The listing builds one solid part. Answer for the finished solid, in the listing's coordinates (mm). Face numbers are marked on the shaded views. A direction names the side the tool comes from. Round coordinates to 2 decimals unless told otherwise and drop trailing zeros. Write each loop counter-clockwise with the first axis right and the second up, starting at its lowest first coordinate (ties: lowest second). Pieces come first, ordered by that corner, then holes. Notation, with made-up numbers: (49.5, 31) - (105.5, 31) arc R21 cw to (105.5, 62) - close; hole circle Ø1 at (-26.5, -3). An arc over 180 degrees is marked (long way). Return JSON: item names as keys, results as strings. Group by question number.
(1) Determine the mould class of the marked faces 1, 2, 3 and 4 for opening direction Y: +Y half, -Y half, draft (parallel to the pull), parting line (faces both ways), or undercut.
(2) Section A-A, the plane x = 27.5 is taken. Write down the section's boundary in (y, z).
(3) Section D-D, the plane z = 12.5 is taken. Write down the section's boundary in (x, y), then the cut area to 3 significant figures.
(4) Find the intervals of material crossed by line 1 along Y through (x, z) = (2.35, 19.8); line 2 along Y through (x, z) = (13.7, 71.9); line 3 along X through (y, z) = (17.5, 18), in increasing order. Write a range as [from, to].
(5) Section B-B, the plane z = 56.4 is taken. Write down the section's boundary in (x, y).
(6) Section C-C, the plane x = 18 is taken. Write down the section's boundary in (y, z), then the cut area to 3 significant figures.
(7) Each of these flat-tipped pins is pushed along its axis until it touches: pin 1 (2.5 mm diameter, centred on y = 11.5, z = 71.9, fed in from -X); pin 2 (5.5 mm diameter, centred on y = 11.5, z = 71.9, fed in from -X); pin 3 (1.8 mm diameter, centred on y = 10, z = 71, fed in from +X). Where does it stop, or does it pass through?
(8) Which of the six approach directions +Z, -Z, +X, -X, +Y, -Y give full straight-line access (tool end or side, diameter ignored) to the marked faces 5, 6 and 7?
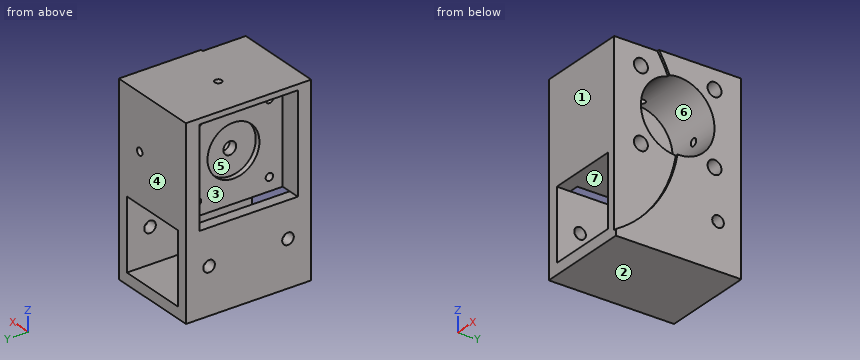
Autodesk Inventor part; units mm, degrees
ref_plane "YZ Plane" through (0, 0, 0) normal (1, 0, 0) x (0, 1, 0)
ref_plane "XZ Plane" through (0, 0, 0) normal (0, 1, 0) x (-1, 0, 0)
ref_plane "XY Plane" through (0, 0, 0) normal (0, 0, 1) x (1, 0, 0)
sketch "Sketch1" plane through (0, 0, 0) normal (0, 0, 1) x (1, 0, 0)
  line L0 (0, 0) -> (40, 0)
  line L1 (40, 0) -> (40, 54)
  line L2 (40, 54) -> (0, 54)
  line L3 (0, 54) -> (0, 0)
  dimension "d0" = 40
  dimension "d1" = 54
extrude "Extrusion1" add sketch "Sketch1" along normal blind 80
sketch "Sketch3" plane through (0, 0, 0) normal (0, -1, 0) x (1, 0, 0)
  line L0 (4.8, 4.8) -> (35.2, 4.8)
  line L1 (35.2, 4.8) -> (35.2, 35.2)
  line L2 (35.2, 35.2) -> (4.8, 35.2)
  line L3 (4.8, 35.2) -> (4.8, 4.8)
  line L4 (0, 0) -> (40, 0)
  line L5 (0, 0) -> (0, 80)
  dimension "d7" = 30.4
  dimension "d8" = 30.4
  dimension "d9" = 4.8
  dimension "d10" = 4.8
extrude "Extrusion2" cut sketch "Sketch3" against normal blind 80
sketch "Sketch4" plane through (0, 0, 0) normal (-1, 0, 0) x (0, 0, 1)
  line L0 (35.2, 0) -> (35.2, 54)
  line L1 (35.2, 5.8) -> (77.6, 5.8)
  line L2 (77.6, 5.8) -> (77.6, 48.2)
  line L3 (77.6, 48.2) -> (35.2, 48.2)
  line L4 (35.2, 48.2) -> (35.2, 5.8)
  line L5 (0, 0) -> (80, 0)
  point P0 (35.2, 48.2)
  dimension "d13" = 42.4
  dimension "d14" = 42.4
  dimension "d15" = 5.8
extrude "Extrusion3" cut sketch "Sketch4" against normal blind 9
sketch "Sketch5" plane through (9, 0, 0) normal (-1, 0, 0) x (0, 0, 1)
  circle A0 centre (71.9, 42.5) radius 1.6
  circle A1 centre (71.9, 11.5) radius 1.6
  circle A2 centre (40.9, 42.5) radius 1.6
  circle A3 centre (40.9, 11.5) radius 1.6
  circle A4 centre (56.4, 27) radius 2.75
  line L0 (71.9, 42.5) -> (71.9, 11.5)
  line L1 (71.9, 11.5) -> (40.9, 11.5)
  line L2 (40.9, 11.5) -> (40.9, 42.5)
  line L3 (40.9, 42.5) -> (71.9, 42.5)
  line L4 (77.6, 48.2) -> (77.6, 5.8)
  line L5 (35.2, 48.2) -> (77.6, 48.2)
  point P0 (0, 0)
  dimension "d18" = 3.2
  dimension "d19" = 31
  dimension "d20" = 31
  dimension "d21" = 5.7
  dimension "d22" = 5.7
  dimension "d23" = 15.5
  dimension "d24" = 15.5
  dimension "d25" = 5.5
extrude "Extrusion4" cut sketch "Sketch5" against normal blind 40 contours A0 L0 L3 | L3 L0 A0 | L3 L2 A2 | A2 L2 L3 | L0 L1 A1 | A1 L1 L0 | L2 L1 A3 | A3 L1 L2 | A4
sketch "Sketch7" plane through (40, 0, 0) normal (1, 0, 0) x (0, 0, -1)
  circle A0 centre (-56.4, 27) radius 15.5
  circle A1 centre (-56.4, 27) radius 2.75
  circle A2 centre (-71.9, 11.5) radius 1.6
  circle A3 centre (-71.9, 11.5) radius 3
  circle A4 centre (-40.9, 11.5) radius 1.6
  circle A5 centre (-40.9, 11.5) radius 3
  circle A6 centre (-40.9, 42.5) radius 1.6
  circle A7 centre (-40.9, 42.5) radius 3
  circle A8 centre (-71.9, 42.5) radius 1.6
  circle A9 centre (-71.9, 42.5) radius 3
  point P0 (0, 0)
  point P1 (-72.8896, 14.2541)
  point P2 (-68.9459, 10.3104)
  point P3 (-43.4541, 10.3104)
  point P4 (-39.5104, 14.2541)
  point P5 (-39.5104, 39.7459)
  point P6 (-43.4541, 43.6896)
  point P7 (-68.9459, 43.6896)
  point P8 (-72.8896, 39.7459)
  dimension "d28" = 31
  dimension "d29" = 6
extrude "Extrusion5" cut sketch "Sketch7" against normal blind 25 contours A0 | A2 | A3 | A4 | A5 | A6 | A7 | A8 | A9
sketch "Sketch8" plane through (0, 0, 80) normal (0, 0, 1) x (1, 0, 0)
  circle A0 centre (18, 27) radius 1.5
  line L0 (40, 54) -> (0, 54)
  line L1 (40, 0) -> (40, 54)
  line L2 (15, 24.25) -> (15, 29.75)
  point P0 (0, 0)
  dimension "d32" = 3
  dimension "d33" = 27
  dimension "d35" = 3
extrude "Extrusion6" cut sketch "Sketch8" against normal blind 10
sketch "Sketch9" plane through (0, 54, 0) normal (0, 1, 0) x (1, 0, 0)
  circle A0 centre (27.5, -56.4) radius 1.6
  line L0 (15, -59.15) -> (15, -53.65)
  line L1 (35.2, -35.2) -> (4.8, -35.2)
  point P0 (0, 0)
  dimension "d38" = 12.5
  dimension "d39" = 3.2
  dimension "d43" = 21.2
extrude "Extrusion7" cut sketch "Sketch9" against normal blind 20
sketch "Sketch10" plane through (40, 0, 0) normal (1, 0, 0) x (0, 0, -1)
  circle A0 centre (-50.2, -27.6494) radius 55
  circle A1 centre (-56.4, 27) radius 2.75
  line L0 (-80, 0) -> (-80, 54)
  point P0 (0, 0)
  point P1 (-59.1239, 26.6218)
  point P2 (-53.6606, 27.2416)
  point P3 (-35.2, 54)
  dimension "d44" = 110
  dimension "d48" = 55
  dimension "d49" = 15
extrude "Extrusion8" cut sketch "Sketch10" against normal blind 1 contours A0 A1 picked at (-46.3005, -46.3752)
sketch "Sketch11" plane through (9, 0, 0) normal (-1, 0, 0) x (0, 0, 1)
  circle A0 centre (56.4, 27) radius 11.2
  circle A1 centre (56.4, 27) radius 2.75
  point P0 (0, 0)
  dimension "d50" = 22.4
extrude "Extrusion9" cut sketch "Sketch11" against normal blind 2.2
sketch "Sketch12" plane through (40, 0, 0) normal (1, 0, 0) x (0, 0, -1)
  circle A0 centre (-19.8, 44) radius 2.5
  line L0 (0, 54) -> (-80, 54)
  point P0 (0, 0)
  point P1 (-4.8, 54)
  dimension "d53" = 15
  dimension "d54" = 5
  dimension "d55" = 10
extrude "Extrusion10" cut sketch "Sketch12" against normal blind 10
sketch "Sketch13" plane through (0, 0, 0) normal (-1, 0, 0) x (0, 0, 1)
  circle A0 centre (19.8, 44) radius 2.5
  circle A1 centre (19.8, 44) radius 2.5
  circle A2 centre (19.8, 10) radius 2.5
  line L0 (0, 54) -> (80, 54)
  line L1 (0, 0) -> (80, 0)
  point P0 (4.8, 54)
  dimension "d58" = 15
  dimension "d59" = 15
  dimension "d62" = 5
  dimension "d63" = 10
extrude "Extrusion11" cut sketch "Sketch13" against normal blind 10
equation "\"d22\" = d21"
properties part number "nema_mount"
Working result:
{
 "1": {"face 1": "-Y half", "face 2": "draft", "face 3": "undercut", "face 4": "+Y half"},
 "2": {"outline": "(0, 0) - (54, 0) - (54, 4.8) - (0, 4.8) - close; (0, 35.2) - (54, 35.2) - (54, 54.8) - (42.42, 54.8) arc R15.5 cw (long way) to (42.42, 58) - (54, 58) - (54, 80) - (0, 80) - close; hole circle Ø6 at (11.5, 40.9); hole circle Ø6 at (11.5, 71.9); hole circle Ø6 at (42.5, 40.9); hole circle Ø6 at (42.5, 71.9)"},
 "3": {"outline": "(0, 0) - (4.8, 0) - (4.8, 54) - (0, 54) - close; (35.2, 0) - (39, 0) - (39, 12.4) - (40, 12.4) - (40, 54) - (35.2, 54) - close", "area": "506 mm^2"},
 "4": {"line 1": "y = [0, 7.5], [12.5, 41.5], [46.5, 54]", "line 2": "y = [0, 9.9], [13.1, 40.9], [44.1, 54]", "line 3": "x = [0, 4.8], [35.2, 40]"},
 "5": {"outline": "(0, 0) - (39, 0) - (39, 11.5) - (15, 11.5) - (15, 24.25) - (11.2, 24.25) - (11.2, 15.8) - (9, 15.8) - (9, 5.8) - (0, 5.8) - close; (0, 48.2) - (9, 48.2) - (9, 38.2) - (11.2, 38.2) - (11.2, 29.75) - (15, 29.75) - (15, 42.5) - (25.9, 42.5) - (25.9, 54) - (0, 54) - close; (29.1, 42.5) - (40, 42.5) - (40, 54) - (29.1, 54) - close"},
 "6": {"outline": "(0, 0) - (54, 0) - (54, 4.8) - (0, 4.8) - close; (0, 35.2) - (54, 35.2) - (54, 80) - (28.5, 80) - (28.5, 71.83) arc R15.5 cw (long way) to (25.5, 71.83) - (25.5, 80) - (0, 80) - close; hole circle Ø6 at (11.5, 40.9); hole circle Ø6 at (11.5, 71.9); hole circle Ø6 at (42.5, 40.9); hole circle Ø6 at (42.5, 71.9)", "area": "1,790 mm^2"},
 "7": {"pin 1": "passes through", "pin 2": "stops at x = 9", "pin 3": "stops at x = 15"},
 "8": {"face 5": "-X", "face 6": "+X", "face 7": "+Y, -Y"}
}
